```python
from build123d import *

# Parameters (mm, degrees)
EXTRUDE_THIN1_DEPTH       = 15
M12_CLEARANCE_SLOT1_D     = 13.5
M12_CLEARANCE_SLOT1_DEPTH = 1


with BuildPart() as part:
    # Sketch1 → Extrude-Thin1 (new body, symmetric)
    with BuildSketch(Plane.XY):
        Polygon((0, 40), (0, 0), (20, 0), (20, -1), (-1, -1), (-1, 40), align=None)
    extrude(amount=EXTRUDE_THIN1_DEPTH, both=True)

    # M12 Clearance Slot1
    with Locations(Plane(origin=(0, 0, 0), x_dir=(1, 0, 0), z_dir=(0, 1, 0))):
        with Locations((10, 0)):
            Hole(M12_CLEARANCE_SLOT1_D / 2, depth=M12_CLEARANCE_SLOT1_DEPTH)


solid = part.part
```
Input: part model. Units: mm. Frame: model coordinates. A direction names the side the tool comes from. Give positions to 0.01 mm unless a question says otherwise; leave off trailing zeros. Order: outer loops, then holes, each group sorted by start corner. A loop starts at its lowest first (then second) coordinate and runs counter-clockwise, first axis right, second up.
1. Reachability of faces 4 (the flat face through (10, 0, 7)), 5 (the flat face through (20, -0.5, 0.2)) from +Z, -Z, +X, -X, +Y, -Y: full face, straight path, thin tool, end or side. Return the list, or none.
Derived:
face 4: +Z, -Z, +X, +Y
face 5: +Z, -Z, +X, +Y, -Y
2. Pin query (flat end, axial travel): pin 1 (12 mm diameter, centred on x = 18, z = -7.5, fed in from +Y); pin 2 (1.5 mm diameter, centred on y = 10.5, z = 4, fed in from +X). Return the tip coordinate at first contact, or that it passes through.
Derived:
pin 1: stops at y = 0
pin 2: stops at x = 0
3. Section C-C on z = -10.5. Return the cut outline in (x, y), and give its area (3 significant figures).
Derived:
outline: (-1, -1) - (20, -1) - (20, 0) - (0, 0) - (0, 40) - (-1, 40) - close
area: 61.0 mm2
4. Section B-B on x = 10. Return the cut outline in (y, z), and give its area (3 significant figures).
Derived:
outline: (-1, -15) - (0, -15) - (0, -6.75) - (-1, -6.75) - close; (-1, 6.75) - (0, 6.75) - (0, 15) - (-1, 15) - close
area: 16.5 mm2
5. Mould query, pull axis X, two halves, no side actions, for faces 1 (the flat face through (-1, 19, 0)), 2 (the flat face through (0, 20, 0)), 3 (the cylindrical face through (3.765, -0.507, 2.585)). Classes: released by +X, released by -X, zero draft, split by the parting line, or undercut.
Derived:
face 1: released by -X
face 2: released by +X
face 3: undercut
6. Section D-D on y = 10. Return the cut outline in (x, z).
Derived:
outline: (-1, -15) - (0, -15) - (0, 15) - (-1, 15) - close
7. Section A-A on z = 0. Return the cut outline in (x, y).
Derived:
outline: (-1, -1) - (3.25, -1) - (3.25, 0) - (0, 0) - (0, 40) - (-1, 40) - close; (16.75, -1) - (20, -1) - (20, 0) - (16.75, 0) - close
8. Material intervals for L1, parallel to Z at x = 10, y = -0.8; L2, parallel to Y at x = 1, z = 7.75, sorted ascending.
Derived:
L1: z = -15 to -6.75, 6.75 to 15
L2: y = -1 to 0
